Autodesk Inventor part; units mm, degrees
ref_plane "YZ Plane" through (0, 0, 0) normal (1, 0, 0) x (0, 1, 0)
ref_plane "XZ Plane" through (0, 0, 0) normal (0, 1, 0) x (-1, 0, 0)
ref_plane "XY Plane" through (0, 0, 0) normal (0, 0, 1) x (1, 0, 0)
sketch "Sketch1" plane through (0, 0, 0) normal (0, 0, 1) x (1, 0, 0)
  line L0 (0, 0) -> (31.75, 0)
  line L1 (31.75, 0) -> (31.75, 31.75)
  line L2 (31.75, 31.75) -> (0, 31.75)
  line L3 (0, 31.75) -> (0, 0)
  dimension "d0" = 31.75
  dimension "d1" = 31.75
extrude "Extrusion1" add sketch "Sketch1" along normal blind 160.3375
sketch "Sketch2" plane through (0, 0, 160.3375) normal (0, 0, 1) x (1, 0, 0)
  circle A0 centre (15.875, 15.875) radius 2.54
  line L0 (31.75, 31.75) -> (0, 31.75)
  line L1 (0, 0) -> (31.75, 0)
  line L2 (0, 31.75) -> (0, 0)
  dimension "d4" = 5.08
  dimension "d5" = 31.75
  dimension "d6" = 15.875
  dimension "d7" = 15.875
extrude "Extrusion2" cut sketch "Sketch2" against normal through all
sketch "Sketch3" plane through (0, 31.75, 0) normal (0, 1, 0) x (1, 0, 0)
  line L0 (31.75, 0) -> (0, 0)
  line L1 (0, 0) -> (0, -160.3375)
  line L2 (31.75, 0) -> (31.75, -160.3375)
  line L3 (31.75, -160.3375) -> (0, -160.3375)
  line L4 (2.032, 0) -> (29.718, 0)
  line L5 (29.718, 0) -> (29.718, -160.3375)
  line L6 (29.718, -160.3375) -> (2.032, -160.3375)
  line L7 (2.032, -160.3375) -> (2.032, 0)
  dimension "d10" = 0
  dimension "d11" = 2.032
  dimension "d12" = 2.032
  dimension "d13" = 0
extrude "Extrusion3" cut sketch "Sketch3" against normal blind 29.718 contours L5 L3 L7 L0
equation "\"d1\" = d0"
equation "\"d6\" = 0.5 * d5"
equation "\"d7\" = d6"
equation "\"d12\" = d11"
properties part number "Claw holding bars"
For this review, take the finished solid that the model builds, in its own axes (mm). A direction names the side the tool comes from. Coordinates: 2 decimals unless noted, no trailing zeros. Write each loop counter-clockwise with the first axis right and the second up, starting at its lowest first coordinate (ties: lowest second). Pieces come first, ordered by that corner, then holes.
(1) Wall thickness on probe 1 along X at (y, z) = (20, 134); probe 2 along Y at (x, z) = (5.5, 101): over which ranges is each line inside the solid? List them lowest first.
(2) Add section A-A on y = 5.5. Give the boundary of the cut face in (x, z), then the cut area to 3 significant figures.
(3) Tool access review of faces 1 (the face through (2.032, 17, 81)), 2 (the face through (31.75, 16, 79)): name each direction out of +Z, -Z, +X, -X, +Y, -Y from which nothing blocks a thin tool from reaching the whole face with its end or side.
(4) The part is to be moulded in two halves that separate along X. For faces 3 (the face through (15.8, 1.8, 160.338)), 4 (the face through (16, 2.032, 79)), 5 (the face through (0, 16, 79)), say which applies: +X half, -X half, draft (parallel to the pull), parting line (faces both ways), or undercut.
(5) For pin 1 Ø1 at (x, z) = (20.5, 125.5) entering from +Y, flat-tipped, find the tip position at first contact; note if it passes through.
(6) Add section C-C on x = 24.5. Give the boundary of the cut face in (y, z), then the cut area to 3 significant figures.
(7) Add section B-B on z = 49. Give the boundary of the cut face in (x, y), then the cut area to 3 significant figures.
Answer sheet:
1. probe 1: x = 0 to 2.03, 29.72 to 31.75
1. probe 2: y = 0 to 2.03
2. outline: (0, 0) - (2.03, 0) - (2.03, 160.34) - (0, 160.34) - close; (29.72, 0) - (31.75, 0) - (31.75, 160.34) - (29.72, 160.34) - close
2. area: 652 mm2
3. face 1: +Z, -Z, +Y
3. face 2: +Z, -Z, +X, +Y, -Y
4. face 3: draft
4. face 4: undercut
4. face 5: -X half
5. pin 1: stops at y = 2.03
6. outline: (0, 0) - (2.03, 0) - (2.03, 160.34) - (0, 160.34) - close
6. area: 326 mm2
7. outline: (0, 0) - (31.75, 0) - (31.75, 31.75) - (29.72, 31.75) - (29.72, 2.03) - (2.03, 2.03) - (2.03, 31.75) - (0, 31.75) - close
7. area: 185 mm2
